```python
from build123d import *

# Parameters (mm, degrees)
F0_W     = 85
F0_H     = 110
F1_DEPTH = 5
F3_DEPTH = 25
F4_R     = 2.225
F5_DEPTH = 25


with BuildPart() as f1:
    # F0 (on Top) → F1 (new body)
    with BuildSketch(Plane.XY):
        Rectangle(F0_W, F0_H)
    extrude(amount=F1_DEPTH)

    # F2 (on face) → F3 (cut)
    with BuildSketch(Plane.XY.offset(5)):
        Polygon((9.925, -20.3), (9.925, 20.3), (-9.925, 20.3), (-9.925, -20.3), (-2.1, -20.3), (-2.1, -25.7), (2.1, -25.7), (2.1, -20.3), align=None)
    extrude(amount=-F3_DEPTH, mode=Mode.SUBTRACT)

    # F4 (on face) → F5 (cut)
    with BuildSketch(Plane.XY.offset(5)):
        with Locations((-5.485, 25.475)):
            Circle(F4_R)
        with Locations((5.485, 25.475)):
            Circle(F4_R)
        with Locations((-5.485, -25.475)):
            Circle(F4_R)
        with Locations((5.485, -25.48)):
            Circle(F4_R)
    extrude(amount=-F5_DEPTH, mode=Mode.SUBTRACT)


solid = f1.part
```
Verification items for the finished model (mm, model axes). A direction names the side the tool comes from. Round coordinates to 2 decimals unless told otherwise and drop trailing zeros. Write each loop counter-clockwise with the first axis right and the second up, starting at its lowest first coordinate (ties: lowest second). Pieces come first, ordered by that corner, then holes.
1. Section check A-A on y = -14. Enter the section's corners in (x, z) (3 decimals).
2. Access from +Z, -Z, +X, -X, +Y, -Y to the whole of each face (thin tool, end or side, straight path). Record for faces 1 (the flat face through (-42.5, -1, 2)), 2 (the flat face through (-9.925, 0, 3)).
3. Scan lines: L1, parallel to X at y = -2, z = 0.9 (3 decimals); L2, parallel to X at y = 23.5, z = 3.95; L3, parallel to X at y = -21, z = 4. Record each from-to range of solid material in increasing order.
4. Draft check along Y on faces 3 (the flat face through (-6, -20.3, 3)), 4 (the flat face through (-1, 55, 2)), 5 (the flat face through (42.5, -1, 2)), 6 (the cylindrical face through (-4.46, -27.45, 2.54)). Enter one of: +Y half, -Y half, draft (parallel to the pull), parting line (faces both ways), or undercut.
5. Section check B-B on z = 1.9. Enter the section's corners in (x, y) (3 decimals).
Answer:
1. outline: (-42.5, 0) - (-9.925, 0) - (-9.925, 5) - (-42.5, 5) - close; (9.925, 0) - (42.5, 0) - (42.5, 5) - (9.925, 5) - close
2. face 1: +Z, -Z, -X, +Y, -Y
2. face 2: +Z, -Z
3. L1: x = -42.5 to -9.925, 9.925 to 42.5
3. L2: x = -42.5 to -6.51, -4.46 to 4.46, 6.51 to 42.5
3. L3: x = -42.5 to -2.1, 2.1 to 42.5
4. face 3: undercut
4. face 4: +Y half
4. face 5: draft
4. face 6: undercut
5. outline: (-42.5, -55) - (42.5, -55) - (42.5, 55) - (-42.5, 55) - close; hole (-9.925, -20.3) - (-2.1, -20.3) - (-2.1, -25.7) - (2.1, -25.7) - (2.1, -20.3) - (9.925, -20.3) - (9.925, 20.3) - (-9.925, 20.3) - close; hole circle Ø4.45 at (-5.485, -25.475); hole circle Ø4.45 at (-5.485, 25.475); hole circle Ø4.45 at (5.485, -25.48); hole circle Ø4.45 at (5.485, 25.475)
